Input: part model. Units: mm. Frame: model coordinates. Face numbers are marked on the shaded views. A direction names the side the tool comes from. Round coordinates to 2 decimals unless told otherwise and drop trailing zeros. Loops run counter-clockwise (first coordinate to the right, second up) from the corner with the lowest first, then second, coordinate; pieces in that order, holes last. Notation, with made-up numbers: (-30.5, 13) -> (6.5, 13) arc R23 cw to (6.5, 26) -> close; hole circle Ø5 at (2, 6). An arc over 180 degrees is marked (long way). Answer as a JSON object with one key per item and string values. Group by question number.
Item 1: Section query B-B on y = 3.3. Return loops of the section in (x, z), and give its area (3 significant figures).
Item 2: Section query D-D on x = -14. Return loops of the section in (y, z), and give its area (3 significant figures).
Item 3: Pin query (flat end, axial travel): pin 1 (2 mm diameter, centred on y = 5, z = -38.5, fed in from +X); pin 2 (3 mm diameter, centred on x = -15, y = 2, fed in from -Z); pin 3 (2 mm diameter, centred on y = 4.5, z = -35, fed in from -X). Return the tip coordinate at first contact, or that it passes through.
Item 4: Draft query along Z for the marked faces 3, 4 and 5. Return one class per face: released by +Z, released by -Z, zero draft, split by the parting line, or undercut.
Item 5: Material intervals for line 1 (X direction, y = 3.5, z = -35); line 2 (Z direction, x = -22, y = 0.5); line 3 (Z direction, x = -36, y = 6.25), sorted ascending. Write a range as [from, to].
Item 6: Section query A-A on z = 10.5. Return loops of the section in (x, y), and give its area (3 significant figures).
Item 7: Section query C-C on z = -36. Return loops of the section in (x, y), and give its area (3 significant figures).
Item 8: Set-up query: the marked faces 1 and 2. Return all of +Z, -Z, +X, -X, +Y, -Y with unobstructed straight access to the full face (end or side cutting, diameter ignored); none if empty.
from build123d import *

# Parameters (mm, degrees)
BOSS_EXTRUDE1_DEPTH = 6.6
SKETCH4_R           = 2
CUT_EXTRUDE1_DEPTH  = 6.6
FILLET1_R           = 2
FILLET2_R           = 0.5
FILLET3_R           = 2
SKETCH5_R           = 2
CUT_EXTRUDE2_DEPTH  = 6.6


with BuildPart() as part:
    # Sketch3 → Boss-Extrude1 (new body)
    with BuildSketch(Plane(origin=(0, 0, 0), x_dir=(1, 0, 0), z_dir=(0, 1, 0))):
        with BuildLine():
            ThreePointArc((-18.186533479, 31.5), (-18.186533479, 10.5), (0, 0))
            Line((0, 0), (0, -3))
            ThreePointArc((0, -3), (-20.888208397, 7.927851418), (-21.186533479, 31.5))
            Line((-21.186533479, 31.5), (-18.186533479, 31.5))
        make_face()
        Polygon((-38.186533479, 42), (-21.186533479, 42), (-21.186533479, 31.5), (-18.186533479, 31.5), (-18.186533479, 45), (-38.186533479, 45), align=None)
        with BuildLine():
            Line((0, -15), (0, -3))
            ThreePointArc((0, -3), (-1.5004505, -3.035167191), (-3, -2.972399899))
            Line((-3, -2.972399899), (-3, -15))
            Line((-3, -15), (0, -15))
        make_face()
    extrude(amount=BOSS_EXTRUDE1_DEPTH)

    # Sketch4 → Cut-Extrude1 (cut)
    with BuildSketch(Plane.XY.offset(-42)):
        with Locations((-32.186533479, 3.3)):
            Circle(SKETCH4_R)
    extrude(amount=-CUT_EXTRUDE1_DEPTH, mode=Mode.SUBTRACT)

    # Fillet1
    fillet1_edges = [part.edges().sort_by_distance(p)[0] for p in [
        (-21.186533479, 3.3, -42),
    ]]
    fillet(fillet1_edges, radius=FILLET1_R)

    # Fillet2
    fillet2_edges = [part.edges().sort_by_distance(p)[0] for p in [
        (-34.186533479, 3.3, -42),
    ]]
    fillet(fillet2_edges, radius=FILLET2_R)

    # Fillet3
    fillet3_edges = [part.edges().sort_by_distance(p)[0] for p in [
        (-3, 3.3, 2.972399899),
    ]]
    fillet(fillet3_edges, radius=FILLET3_R)

    # Sketch5 → Cut-Extrude2 (cut)
    with BuildSketch(Plane.ZY.offset(3)):
        with Locations((10.5, 3.3)):
            Circle(SKETCH5_R)
    extrude(amount=-CUT_EXTRUDE2_DEPTH, mode=Mode.SUBTRACT)


solid = part.part
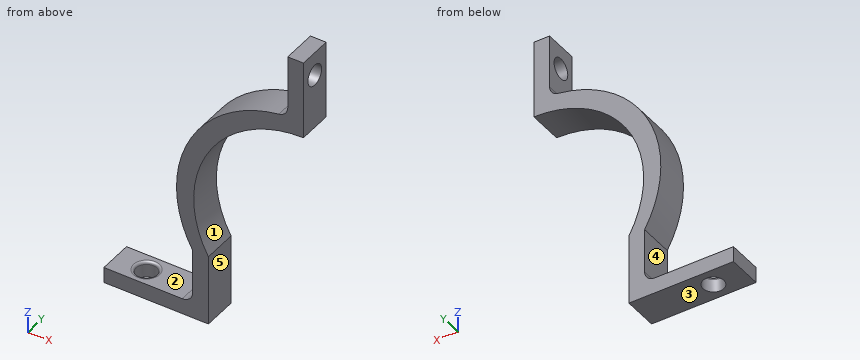
Solved:
{
 "1": {"outline": "(-38.19, -45) -> (-34.19, -45) -> (-34.19, -42.5) arc R0.5 ccw to (-34.69, -42) -> (-38.19, -42) -> close; (-30.19, -45) -> (-18.19, -45) -> (-18.19, -31.5) arc R21 cw to (0, 0) -> (0, 8.5) -> (-3, 8.5) -> (-3, 4.76) arc R2 cw to (-4.7, 2.78) arc R23 ccw to (-21.19, -31.5) -> (-21.19, -40) arc R2 cw to (-23.19, -42) -> (-29.69, -42) arc R0.5 ccw to (-30.19, -42.5) -> close; (-3, 12.5) -> (0, 12.5) -> (0, 15) -> (-3, 15) -> close", "area": "261 mm²"},
 "2": {"outline": "(0, -5.35) -> (6.6, -5.35) -> (6.6, -0.8) -> (0, -0.8) -> close", "area": "30.0 mm²"},
 "3": {"pin 1": "x = -18.19", "pin 2": "z = -8.01", "pin 3": "x = -21.19"},
 "4": {"face 3": "released by -Z", "face 4": "undercut", "face 5": "zero draft"},
 "5": {"line 1": "[-21.19, -18.19]", "line 2": "[-45, -41.61], [-29.97, -9.96]", "line 3": "[-45, -42]"},
 "6": {"outline": "(-3, 0) -> (0, 0) -> (0, 1.3) -> (-3, 1.3) -> close; (-3, 5.3) -> (0, 5.3) -> (0, 6.6) -> (-3, 6.6) -> close", "area": "7.80 mm²"},
 "7": {"outline": "(-21.19, 0) -> (-18.19, 0) -> (-18.19, 6.6) -> (-21.19, 6.6) -> close", "area": "19.8 mm²"},
 "8": {"face 1": "+X, +Y, -Y", "face 2": "-X, +Y, -Y"}
}
